Job drawing, mm, ordinate dimensions from the low corner. One solid piece. A direction names the side the tool comes from. Round coordinates to 2 decimals unless told otherwise and drop trailing zeros. Loops run counter-clockwise (first coordinate to the right, second up) from the corner with the lowest first, then second, coordinate; pieces in that order, holes last. Notation, with made-up numbers: M 16,76 L 45,76 A14 ccw 45,81 Z; hole C -17,35 d8. An arc over 180 degrees is marked long. Write each question's results on one line, items separated by ' | '. Start each with the question number.
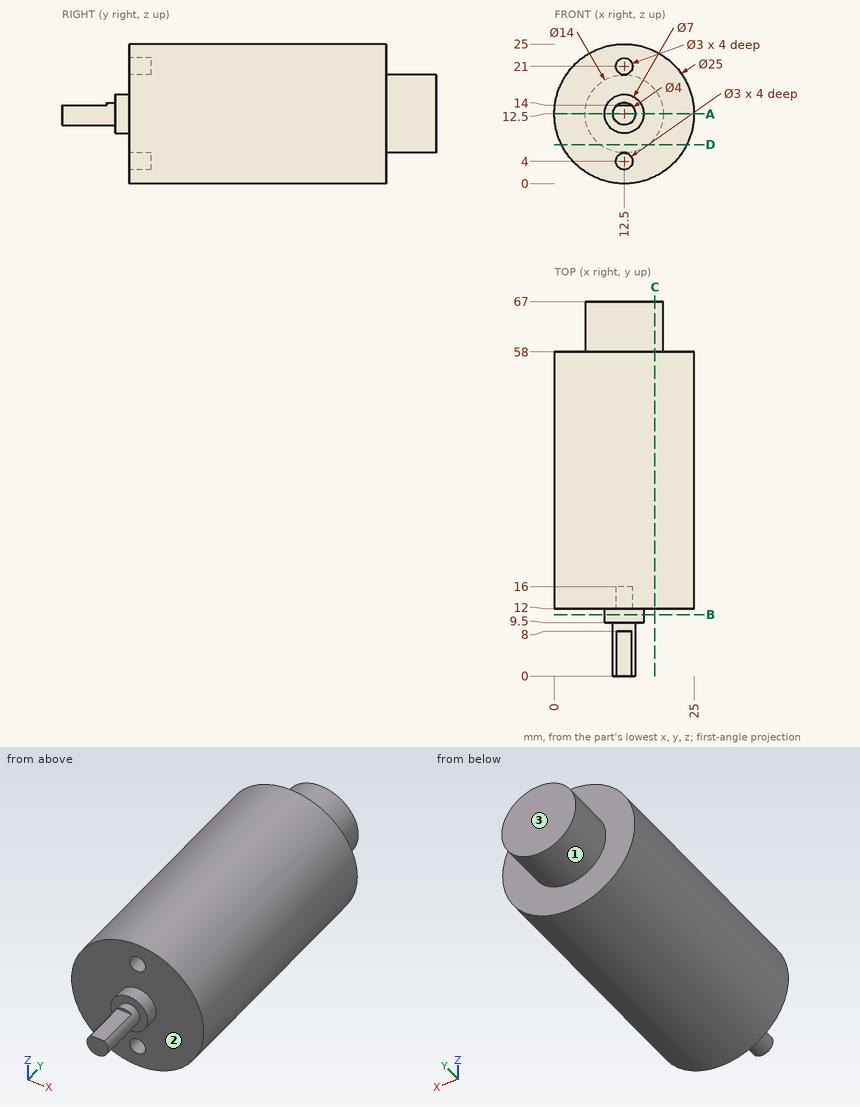
Item 1: Saw through at D-D, the plane z = 7. Give the cut face in (x, y), then the cut area to 3 significant figures.
Item 2: Saw through at B-B, the plane y = 11. Give the cut face in (x, z).
Item 3: Drill centre lines: line 1 along Z through (x, y) = (12.5, 12.9); line 2 along Z through (x, y) = (13, 12.5); line 3 along Y through (x, z) = (21.75, 18.5). Where is each one in solid material? Low to high. Write a range as [from, to].
Item 4: Tool access for the marked faces 1, 2 and 3: list every direction of +Z, -Z, +X, -X, +Y, -Y with a clear straight run to the whole face (end or side of a thin tool).
Item 5: Saw through at A-A, the plane z = 12.5. Give the cut face in (x, y).
Item 6: Drop flat-ended pins along their axis: pin 1 (0.9 mm diameter, centred on x = 12, z = 20.5, fed in from -Y); pin 2 (4 mm diameter, centred on x = 5.5, z = 11.5, fed in from -Y); pin 3 (8 mm diameter, centred on y = 31, z = 3, fed in from +X) (3 decimals). Give the stop position or say it passes through.
Item 7: Saw through at C-C, the plane x = 18. Give the cut face in (y, z), then the cut area to 3 significant figures.
Working result:
1) outline: M 1.28,12 L 23.72,12 L 23.72,58 L 16.83,58 L 16.83,67 L 8.17,67 L 8.17,58 L 1.28,58 Z | area: 1,110 mm²
2) outline: C 12.5,12.5 d7
3) line 1: z = [0, 2.5], [5.5, 19.5], [22.5, 25] | line 2: z = [0.01, 2.59], [5.41, 19.59], [22.41, 24.99] | line 3: y = [12, 58]
4) face 1: +Y | face 2: -Y | face 3: +Z, -Z, +X, -X, +Y
5) outline: M 0,12 L 9,12 L 9,9.5 L 10.5,9.5 L 10.5,0 L 14.5,0 L 14.5,9.5 L 16,9.5 L 16,12 L 25,12 L 25,58 L 19.5,58 L 19.5,67 L 5.5,67 L 5.5,58 L 0,58 Z
6) pin 1: stops at y = 16 | pin 2: stops at y = 12 | pin 3: stops at x = 23.725
7) outline: M 12,1.28 L 58,1.28 L 58,8.17 L 67,8.17 L 67,16.83 L 58,16.83 L 58,23.72 L 12,23.72 Z | area: 1,110 mm²
